Work out the finished part from the listing and answer in its coordinate system (mm). Face numbers are marked on the shaded views. A direction names the side the tool comes from. Round coordinates to 2 decimals unless told otherwise and drop trailing zeros. Write each loop counter-clockwise with the first axis right and the second up, starting at its lowest first coordinate (ties: lowest second). Pieces come first, ordered by that corner, then holes.
1. Find section A-A (z = 60.5). Write down the section's boundary in (x, y).
2. Flat-ended cylindrical pins translate along their axes: pin 1 Ø4 at (x, z) = (5.5, 61) entering from -Y; pin 2 Ø10 at (x, y) = (-4, -37.5) entering from +Z; pin 3 Ø6 at (x, y) = (28.5, -35) entering from +Z; pin 4 Ø2 at (x, y) = (0.5, -37.5) entering from +Z. Find the tip coordinate at first contact, or state that the pin passes through.
3. Find section C-C (y = -18). Write down the section's boundary in (x, z).
4. Find section D-D (z = 7). Write down the section's boundary in (x, y).
5. Straight lines are drawn through the part: probe 1 along Y at (x, z) = (43.5, 54); probe 2 along X at (y, z) = (-20.5, 61); probe 3 along Z at (x, y) = (23.5, 8). For each, find the intervals that lie inside material, in ascending order.
6. A tool of negligible diameter and unlimited length cuts with its end or side. For the marked faces 1 and 2, from which of +Z, -Z, +X, -X, +Y, -Y can it reach the whole face along a straight path? Write none if from no direction.
7. Find section B-B (x = 34). Write down the section's boundary in (y, z), and give its area (3 significant figures).
```python
from build123d import *

# Parameters (mm, degrees)
F0_W     = 95.863237977
F0_H     = 52.7086667717
F1_DEPTH = 78.232
F2_R     = 31.7719269524
F2_R_2   = 26.0233800566
F3_DEPTH = 16.764
F4_DEPTH = 137.668


with BuildPart() as f1:
    # F0 (on Top) → F1 (new body)
    with BuildSketch(Plane.XY):
        with Locations((11.8457712233, -3.3831223845)):
            Rectangle(F0_W, F0_H)
    extrude(amount=F1_DEPTH)

    # F2 (on face) → F3 (join)
    with BuildSketch(Plane.XZ.offset(29.7374557704)):
        with Locations((12.4230552465, 37.5379212201)):
            Circle(F2_R)
        with Locations((12.4230552465, 37.5379212201)):
            Circle(F2_R_2, mode=Mode.SUBTRACT)
    extrude(amount=F3_DEPTH)

    # F4 (cut): a face of the model
    f4_faces = [f1.faces().sort_by_distance(p)[0] for p in [
        (12.4230552465, -29.7374557704, 37.5379212201),
    ]]
    extrude(f4_faces, amount=-F4_DEPTH, mode=Mode.SUBTRACT)


solid = f1.part
```
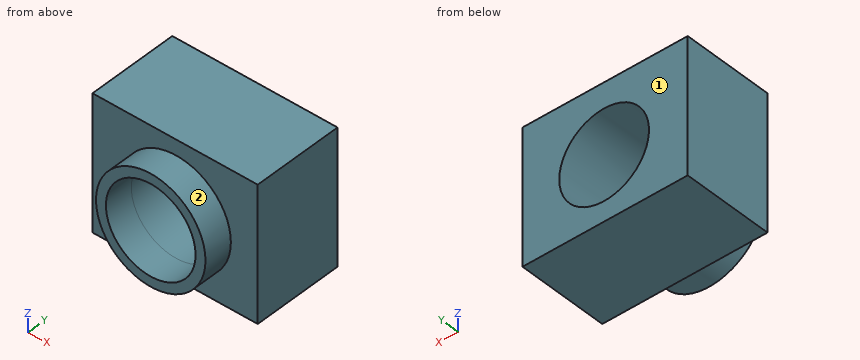
Worked answers:
1. outline: (-36.09, -29.74) - (-9.54, -29.74) - (-9.54, -46.5) - (0.18, -46.5) - (0.18, 22.97) - (-36.09, 22.97) - close; (24.67, -46.5) - (34.38, -46.5) - (34.38, -29.74) - (59.78, -29.74) - (59.78, 22.97) - (24.67, 22.97) - close
2. pin 1: stops at y = -46.5
2. pin 2: stops at z = 67.19
2. pin 3: stops at z = 66.49
2. pin 4: stops at z = 67.37
3. outline: (-36.09, 0) - (59.78, 0) - (59.78, 78.23) - (-36.09, 78.23) - close; hole circle Ø52.05 at (12.42, 37.54)
4. outline: (-36.09, -29.74) - (3.65, -29.74) - (3.65, -46.5) - (21.19, -46.5) - (21.19, -29.74) - (59.78, -29.74) - (59.78, 22.97) - (-36.09, 22.97) - close
5. probe 1: y = -29.74 to 22.97
5. probe 2: x = -36.09 to 1.16, 23.68 to 59.78
5. probe 3: z = 0 to 13.99, 61.09 to 78.23
6. face 1: +Z, -Z, +X, -X, +Y
6. face 2: -Y
7. outline: (-46.5, 14.22) - (-29.74, 14.22) - (-29.74, 0) - (22.97, 0) - (22.97, 22.99) - (-46.5, 22.99) - close; (-46.5, 52.09) - (22.97, 52.09) - (22.97, 78.23) - (-29.74, 78.23) - (-29.74, 60.86) - (-46.5, 60.86) - close
7. area: 2,880 mm2
